Read the model definition and answer for the solid it produces. Units are mm, in the model's axes. Face numbers are marked on the shaded views. A direction names the side the tool comes from. Round coordinates to 2 decimals unless told otherwise and drop trailing zeros. Write each loop counter-clockwise with the first axis right and the second up, starting at its lowest first coordinate (ties: lowest second). Pieces come first, ordered by that corner, then holes. Notation, with made-up numbers: (47, -20.75) - (88, -20.75) arc R26 ccw to (88, 7.25) - close; hole circle Ø8 at (22.25, 17). An arc over 180 degrees is marked (long way). One line per item, written item: value. Start each with the question number.
(1) A cutting plane is placed at D-D, the plane y = -79. Determine the outline of the cut face in (x, z).
(2) A cutting plane is placed at B-B, the plane x = 0. Determine the outline of the cut face in (y, z), plus the area to 3 significant figures.
(3) For the marked faces 1, 2, 3, 4 and 5, determine the directions among +Z, -Z, +X, -X, +Y, -Y from which every point of the face is accessible in a straight line to the end or side of a thin tool.
(4) A cutting plane is placed at C-C, the plane y = -92. Determine the outline of the cut face in (x, z).
(5) Find the intervals of material crossed by L1, parallel to X at y = 9, z = -50; L2, parallel to X at y = -15, z = -41.5; L3, parallel to Y at x = 26, z = -35, in increasing order.
(6) Flat-ended cylindrical pins translate along their axes: pin 1 Ø18 at (x, z) = (-4, 64) entering from -Y; pin 2 Ø12 at (x, z) = (-70, -45) entering from -Y; pin 3 Ø4 at (y, z) = (12, 35) entering from -X. Find the tip coordinate at first contact, or state that the pin passes through.
(7) A cutting plane is placed at A-A, the plane z = -35. Determine the outline of the cut face in (x, y).
(8) The mould has two halves that part along X. Classify the marked faces 6, 7, 8 and 9: +X half, -X half, draft (parallel to the pull), parting line (faces both ways), or undercut.
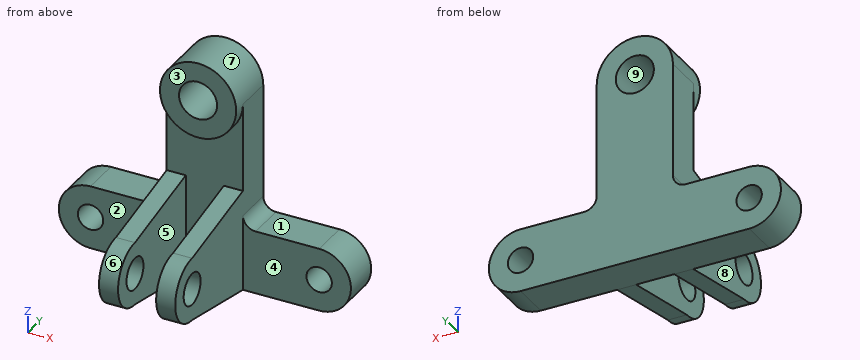
Solid Edge part; units mm, degrees
sketch "Sketch1" plane through (0, 0, 0) normal (0, -1, 0) x (1, 0, 0)
  line L0 (30, -75) -> (30, 75)
  line L1 (-30, 75) -> (-30, -75)
  line L2 (-30, -75) -> (30, -75)
  arc A0 (-30, 75) -> (30, 75) centre (0, 75) cw
extrude "Protrusion1" add sketch "Sketch1" against normal blind 30
sketch "Sketch2" plane through (0, 0, 15) normal (0, -1, 0) x (1, 0, 0)
  circle A0 centre (0, 60) radius 30
extrude "ExtrudedProtrusion_2" add sketch "Sketch2" along normal blind 10
sketch "Sketch3" plane through (0, -10, 75) normal (0, -1, 0) x (1, 0, 0)
  circle A0 centre (0, 0) radius 15
extrude "ExtrudedCutout_1" cut sketch "Sketch3" against normal blind 40
sketch "Sketch4" plane through (-30, 15, 0) normal (-1, 0, 0) x (0, 0, 1)
  line L0 (5, -15) -> (-10, -90)
  line L1 (-75, -15) -> (-60, -90)
  line L2 (5, -15) -> (-75, -15)
  arc A0 (-10, -90) -> (-60, -90) centre (-35, -90) cw
extrude "ExtrudedProtrusion_3" add sketch "Sketch4" against normal blind 15
sketch "Sketch5" plane through (-30, 15, 0) normal (-1, 0, 0) x (0, 0, 1)
  circle A0 centre (-35, -90) radius 12.5
extrude "ExtrudedCutout_2" cut sketch "Sketch5" against normal blind 15
sketch "Sketch6" plane through (30, 15, 0) normal (1, 0, 0) x (0, 0, -1)
  line L0 (60, -90) -> (75, -15)
  line L1 (-5, -15) -> (75, -15)
  line L2 (10, -90) -> (-5, -15)
  arc A0 (60, -90) -> (10, -90) centre (35, -90) cw
extrude "ExtrudedProtrusion_4" add sketch "Sketch6" against normal blind 15
sketch "Sketch7" plane through (-30, 15, 0) normal (-1, 0, 0) x (0, 0, 1)
  circle A0 centre (-35, -90) radius 12.5
extrude "Cutout1" cut sketch "Sketch7" against normal up to vertex (60 mm away)
sketch "Sketch8" plane through (0, 0, 0) normal (0, -1, 0) x (0, 0, -1)
  line L0 (25, 40) -> (25, 90)
  line L1 (75, 90) -> (75, 30)
  line L2 (75, 30) -> (25, 30)
  line L3 (25, 30) -> (15, 30)
  arc A0 (25, 90) -> (75, 90) centre (50, 90) cw
  arc A1 (25, 40) -> (15, 30) centre (15, 40) cw
extrude "ExtrudedProtrusion_5" add sketch "Sketch8" against normal blind 30
sketch "Sketch9" plane through (0, 0, 0) normal (0, -1, 0) x (0, 0, -1)
  circle A0 centre (50, 90) radius 10
extrude "ExtrudedCutout_4" cut sketch "Sketch9" against normal blind 30
sketch "Sketch10" plane through (0, 0, 0) normal (0, -1, 0) x (0, 0, -1)
  line L0 (25, -40) -> (25, -90)
  line L1 (75, -90) -> (75, -30)
  line L2 (75, -30) -> (25, -30)
  line L3 (25, -30) -> (15, -30)
  arc A0 (75, -90) -> (25, -90) centre (50, -90) cw
  arc A1 (15, -30) -> (25, -40) centre (15, -40) cw
extrude "ExtrudedProtrusion_6" add sketch "Sketch10" against normal blind 30
sketch "Sketch11" plane through (0, 0, 0) normal (0, -1, 0) x (0, 0, -1)
  circle A0 centre (50, -90) radius 10
extrude "ExtrudedCutout_5" cut sketch "Sketch11" against normal blind 30
Here are the results:
1. outline: (-30, -59.68) - (-15, -59.68) - (-15, -46.84) - (-30, -46.84) - close; (-30, -23.16) - (-15, -23.16) - (-15, -10.32) - (-30, -10.32) - close; (15, -59.68) - (30, -59.68) - (30, -46.84) - (15, -46.84) - close; (15, -23.16) - (30, -23.16) - (30, -10.32) - (15, -10.32) - close
2. outline: (-10, 45) - (0, 45) - (0, -75) - (30, -75) - (30, 60) - (-10, 60) - close; (-10, 90) - (30, 90) - (30, 105) - (-10, 105) - close
2. area: 4,800 mm²
3. face 1: +Z, +X, +Y, -Y
3. face 2: +Z, -Z, -X, -Y
3. face 3: +Z, +X, -X, -Y
3. face 4: +Z, -Z, +X, -Y
3. face 5: -Z, -Y
4. outline: (-30, -53.33) - (-15, -53.33) - (-15, -16.67) - (-30, -16.67) - close; (15, -53.33) - (30, -53.33) - (30, -16.67) - (15, -16.67) - close
5. L1: -115 to -100, -80 to 80, 100 to 115
5. L2: -30 to -15, 15 to 30
5. L3: -100 to -87.5, -62.5 to 30
6. pin 1: y = -10
6. pin 2: y = 0
6. pin 3: x = -30
7. outline: (-110, 0) - (-30, 0) - (-30, -62.5) - (-15, -62.5) - (-15, 0) - (15, 0) - (15, -62.5) - (30, -62.5) - (30, 0) - (110, 0) - (110, 30) - (-110, 30) - close; (-30, -100) - (-15, -100) - (-15, -87.5) - (-30, -87.5) - close; (15, -100) - (30, -100) - (30, -87.5) - (15, -87.5) - close
8. face 6: draft
8. face 7: parting line
8. face 8: -X half
8. face 9: undercut
